Drawing for the job (mm, zero at the part's lowest x, y, z). Give positions to 0.01 mm unless a question says otherwise; leave off trailing zeros. Order: outer loops, then holes, each group sorted by start corner. A loop starts at its lowest first (then second) coordinate and runs counter-clockwise, first axis right, second up. Notation, with made-up numbers: (48, 81) - (89, 81) arc R25 ccw to (89, 107) - close; hole circle Ø10 at (2, 78). An arc over 180 degrees is marked (long way). Write each question's results on one line, items separated by ' | '. Start each with the question number.
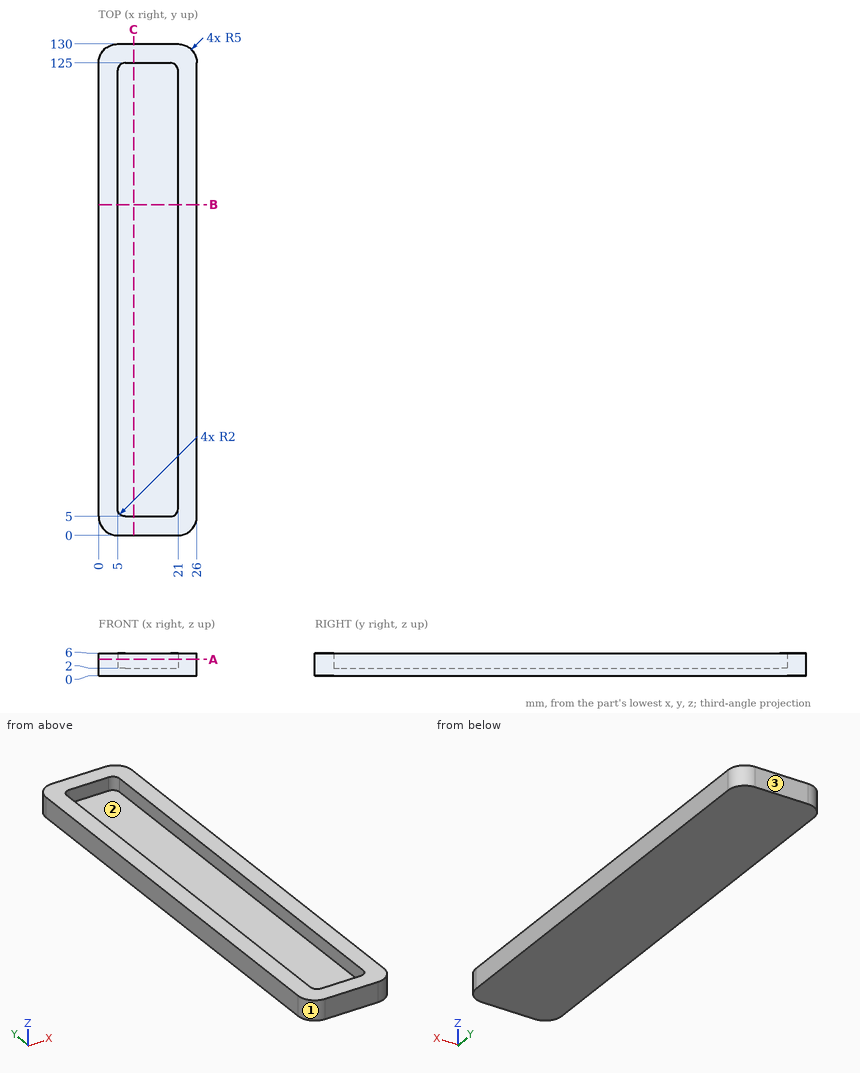
Item 1: Flat gauge pins, fed straight in: pin 1 Ø2 at (x, z) = (16, 4.5) entering from -Y; pin 2 Ø10 at (x, y) = (15.5, 45) entering from +Z. Where does each tip first touch, or does it go through?
Item 2: Two-plate mould, pull along X, no slides. Class the marked faces 1, 2 and 3: +X half, -X half, draft (parallel to the pull), parting line (faces both ways), or undercut.
Item 3: Cut at A-A, the plane z = 4.4. List the corners of the cut face in (x, y).
Item 4: Probe line 1 along X through (y, z) = (14.5, 3.7); line 2 along Y through (x, z) = (7.25, 3.4); line 3 along Z through (x, y) = (13.75, 21). List the from-to ranges inside material, lowest first. Write a range as from..to.
Item 5: Cut at C-C, the plane x = 9.25. List the corners of the cut face in (y, z).
Item 6: Cut at B-B, the plane y = 87.5. List the corners of the cut face in (x, z), then the cut area to 3 significant figures.
Values found:
1) pin 1: stops at y = 0 | pin 2: stops at z = 2
2) face 1: -X half | face 2: undercut | face 3: draft
3) outline: (0, 5) arc R5 ccw to (5, 0) - (21, 0) arc R5 ccw to (26, 5) - (26, 125) arc R5 ccw to (21, 130) - (5, 130) arc R5 ccw to (0, 125) - close; hole (5, 7) arc R2 ccw to (7, 5) - (19, 5) arc R2 ccw to (21, 7) - (21, 123) arc R2 ccw to (19, 125) - (7, 125) arc R2 ccw to (5, 123) - close
4) line 1: x = 0..5, 21..26 | line 2: y = 0..5, 125..130 | line 3: z = 0..2
5) outline: (0, 0) - (130, 0) - (130, 6) - (125, 6) - (125, 2) - (5, 2) - (5, 6) - (0, 6) - close
6) outline: (0, 0) - (26, 0) - (26, 6) - (21, 6) - (21, 2) - (5, 2) - (5, 6) - (0, 6) - close | area: 92.0 mm2
